Read the model definition and answer for the solid it produces. Units are mm, in the model's axes. A direction names the side the tool comes from. Round coordinates to 2 decimals unless told otherwise and drop trailing zeros. Order: outer loops, then holes, each group sorted by start corner. A loop starts at its lowest first (then second) coordinate and runs counter-clockwise, first axis right, second up. Notation, with made-up numbers: (-5, -5.75) - (39, -5.75) arc R13 cw to (39, 13.25) - close; hole circle Ø7 at (13, 72.5). An arc over 180 degrees is marked (long way). Answer as a JSON object with one key per item and string values. Group by question number.
Q1. The mould has two halves that part along Z. Classify faces 1 (the flat face through (9, 8, -9)), 2 (the flat face through (17, 4, 6.5)), 3 (the flat face through (-16.5, 4, 0)): pulls with the +Z half, pulls with the -Z half, needs draft (parallel to the pull), parting line crosses it, or undercut.
Q2. A cutting plane is placed at D-D on x = 16.5. Determine the outline of the cut face in (y, z), and give its area (3 significant figures).
Q3. Consider line 1 (Y direction, x = -16.5, z = 10.25); line 2 (X direction, y = 1.2, z = 0); line 3 (Z direction, x = -3, y = 0.75). Determine where each line is inside the solid, lowest interval first.
Q4. Given pin 1 Ø7 at (x, z) = (-3, 4.5) entering from +Y; pin 2 Ø2 at (x, y) = (16.5, 4) entering from +Z; pin 3 Ø2 at (x, y) = (-16.5, 4) entering from -Z, each flat-ended and moving along its own axis, determine where each tip first touches the part or whether it passes through.
Q5. A tool of negligible diameter and unlimited length cuts with its end or side. For faces 4 (the flat face through (-20.5, 4, -10)), 5 (the flat face through (-18, 4, 5)), 6 (the cylindrical face through (15.923, 5.109, 10.049)), 7 (the flat face through (-17, 4, -6.5)), 8 (the flat face through (4, 2, 9)), from which of +Z, -Z, +X, -X, +Y, -Y can it reach the whole face along a straight path? Write none if from no direction.
Q6. A cutting plane is placed at C-C on z = 0. Determine the outline of the cut face in (x, y), and give its area (3 significant figures).
Q7. A cutting plane is placed at B-B on y = 7.5. Determine the outline of the cut face in (x, z).
Q8. A cutting plane is placed at A-A on x = 0. Determine the outline of the cut face in (y, z), and give its area (3 significant figures).
```python
from build123d import *

# Parameters (mm, degrees)
SKETCH_1_W          = 41
SKETCH_1_H          = 27
SKETCH_1_R          = 9.5
EXTRUDE_1_DEPTH     = 8
SKETCH_2_R          = 12
CUT_EXTRUDE_1_DEPTH = 6
CUT_EXTRUDE_2_DEPTH = 8
SKETCH_4_R          = 1.25
CUT_EXTRUDE_3_DEPTH = 7
SKETCH_5_R          = 1.25
CUT_EXTRUDE_4_DEPTH = 7


with BuildPart() as part:
    # Эскиз1 → Бобышка-Вытянуть1 (new body)
    with BuildSketch(Plane(origin=(0, 0, 0), x_dir=(1, 0, 0), z_dir=(0, 1, 0))):
        Rectangle(SKETCH_1_W, SKETCH_1_H)
        with Locations(Location((0, 0, 0), (0, 0, 270))):  # turned: the seam where the file's is
            Circle(SKETCH_1_R, mode=Mode.SUBTRACT)
    extrude(amount=EXTRUDE_1_DEPTH)

    # Эскиз2 → Вырез-Вытянуть1 (cut)
    with BuildSketch(Plane(origin=(0, 8, 0), x_dir=(1, 0, 0), z_dir=(0, 1, 0))):
        with Locations(Location((0, 0, 0), (0, 0, 270))):  # turned: the seam where the file's is
            Circle(SKETCH_2_R)
    extrude(amount=-CUT_EXTRUDE_1_DEPTH, mode=Mode.SUBTRACT)

    # Эскиз3 → Вырез-Вытянуть2 (cut)
    with BuildSketch(Plane(origin=(0, 8, 0), x_dir=(1, 0, 0), z_dir=(0, 1, 0))):
        Polygon((-20.5, 7.5), (-16.5, 3.5), (-16.5, -3.5), (-20.5, -7.5), align=None)
    extrude(amount=-CUT_EXTRUDE_2_DEPTH, mode=Mode.SUBTRACT)

    # Эскиз4 → Вырез-Вытянуть3 (cut)
    with BuildSketch(Plane.XY.offset(13.5)):
        with Locations((-16.5, 4)):
            Circle(SKETCH_4_R)
        with Locations(Location((16.5, 4, 0), (0, 0, 180))):  # turned: the seam where the file's is
            Circle(SKETCH_4_R)
    extrude(amount=-CUT_EXTRUDE_3_DEPTH, mode=Mode.SUBTRACT)

    # Эскиз5 → Вырез-Вытянуть4 (cut)
    with BuildSketch(Plane(origin=(0, 0, -13.5), x_dir=(-1, 0, 0), z_dir=(0, 0, -1))):
        with Locations((-16.5, 4)):
            Circle(SKETCH_5_R)
        with Locations(Location((16.5, 4, 0), (0, 0, 180))):  # turned: the seam where the file's is
            Circle(SKETCH_5_R)
    extrude(amount=-CUT_EXTRUDE_4_DEPTH, mode=Mode.SUBTRACT)


solid = part.part
```
Result set:
{
 "1": {"face 1": "needs draft", "face 2": "pulls with the +Z half", "face 3": "undercut"},
 "2": {"outline": "(0, -13.5) - (2.75, -13.5) - (2.75, -6.5) - (5.25, -6.5) - (5.25, -13.5) - (8, -13.5) - (8, 13.5) - (5.25, 13.5) - (5.25, 6.5) - (2.75, 6.5) - (2.75, 13.5) - (0, 13.5) - close", "area": "181 mm²"},
 "3": {"line 1": "y = 0 to 2.75, 5.25 to 8", "line 2": "x = -16.5 to -9.5, 9.5 to 20.5", "line 3": "z = -13.5 to -9.01, 9.01 to 13.5"},
 "4": {"pin 1": "passes through", "pin 2": "stops at z = 6.5", "pin 3": "stops at z = -6.5"},
 "5": {"face 4": "+Z, -Z, -X, +Y, -Y", "face 5": "-X, +Y, -Y", "face 6": "+Z", "face 7": "-Z", "face 8": "+Y"},
 "6": {"outline": "(-16.5, 0) - (-9.5, 0) - (-9.5, 2) - (-12, 2) - (-12, 8) - (-16.5, 8) - close; (9.5, 0) - (20.5, 0) - (20.5, 8) - (12, 8) - (12, 2) - (9.5, 2) - close", "area": "114 mm²"},
 "7": {"outline": "(-20.5, -13.5) - (20.5, -13.5) - (20.5, 13.5) - (-20.5, 13.5) - (-20.5, 7.5) - (-16.5, 3.5) - (-16.5, -3.5) - (-20.5, -7.5) - close; hole circle Ø24 at (0, 0)"},
 "8": {"outline": "(0, -13.5) - (8, -13.5) - (8, -12) - (2, -12) - (2, -9.5) - (0, -9.5) - close; (0, 9.5) - (2, 9.5) - (2, 12) - (8, 12) - (8, 13.5) - (0, 13.5) - close", "area": "34.0 mm²"}
}
